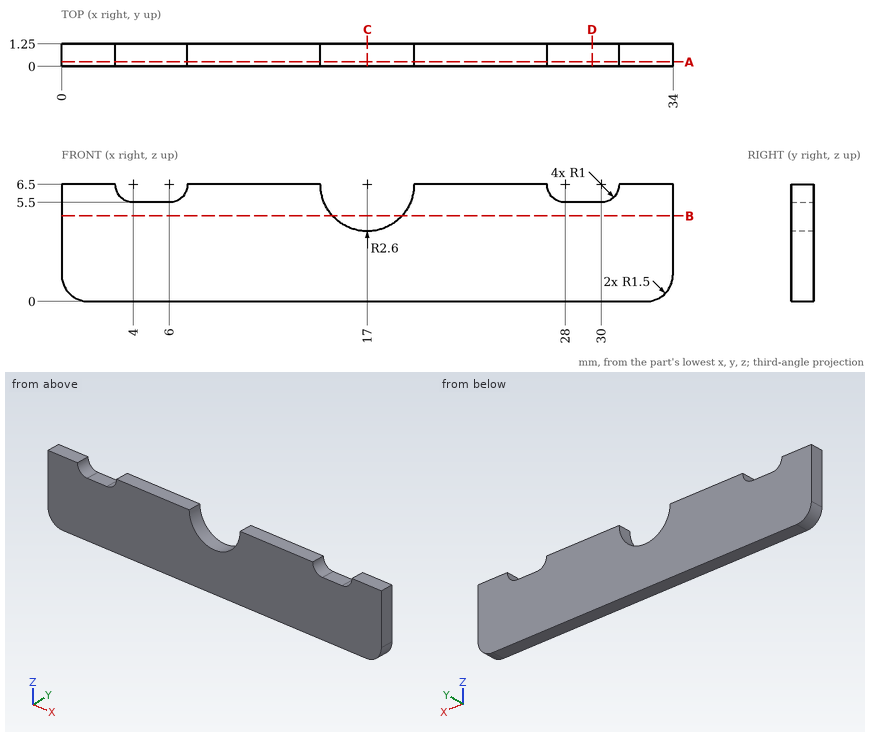
The drawing under review shows one solid part. Ordinate dimensions are in mm from its lowest x, y, z. Coordinates: 2 decimals unless noted, no trailing zeros. Write each loop counter-clockwise with the first axis right and the second up, starting at its lowest first coordinate (ties: lowest second). Pieces come first, ordered by that corner, then holes. Notation, with made-up numbers: (83.25, -34) - (122.25, -34) arc R5 cw to (122.25, -26) - close; hole circle Ø4 at (1, -34.5). An arc over 180 degrees is marked (long way). Answer in a Markdown table with one row per item. Add a question column.
Q1. We need section A-A, the plane y = 0.25. State the section outline as (x, z) points.
Q2. We need section D-D, the plane x = 29.5. State the section outline as (y, z) points.
Q3. For probe 1 along X at (y, z) = (0.4, 6.25); probe 2 along X at (y, z) = (0.3, 6); probe 3 along Z at (x, y) = (28, 0.2), list the stretches that pass through material, from the lowest coordinate up.
Q4. We need section B-B, the plane z = 4.75. State the section outline as (x, y) points.
Q5. We need section C-C, the plane x = 17. State the section outline as (y, z) points, and give its area (4 significant figures).
Answer list:
| question | item | result |
|---|---|---|
| 1 | outline | (0, 1.5) arc R1.5 ccw to (1.5, 0) - (32.5, 0) arc R1.5 ccw to (34, 1.5) - (34, 6.5) - (31, 6.5) arc R1 cw to (30, 5.5) - (28, 5.5) arc R1 cw to (27, 6.5) - (19.6, 6.5) arc R2.6 cw to (14.4, 6.5) - (7, 6.5) arc R1 cw to (6, 5.5) - (4, 5.5) arc R1 cw to (3, 6.5) - (0, 6.5) - close |
| 2 | outline | (0, 0) - (1.25, 0) - (1.25, 5.5) - (0, 5.5) - close |
| 3 | probe 1 | x = 0 to 3.03, 6.97 to 14.41, 19.59 to 27.03, 30.97 to 34 |
| 3 | probe 2 | x = 0 to 3.13, 6.87 to 14.45, 19.55 to 27.13, 30.87 to 34 |
| 3 | probe 3 | z = 0 to 5.5 |
| 4 | outline | (0, 0) - (15.08, 0) - (15.08, 1.25) - (0, 1.25) - close; (18.92, 0) - (34, 0) - (34, 1.25) - (18.92, 1.25) - close |
| 5 | outline | (0, 0) - (1.25, 0) - (1.25, 3.9) - (0, 3.9) - close |
| 5 | area | 4.875 mm2 |
